```python
from build123d import *

# Parameters (mm, degrees)
SKETCH_1_W                   = 80
SKETCH_1_H                   = 40
EXTRUDE_1_DEPTH              = 20
HOLE_WIZARD_M3_1_D           = 4
HOLE_WIZARD_M3_1_CBORE_D     = 7
HOLE_WIZARD_M3_1_CBORE_DEPTH = 7
SKETCH_6_W                   = 7
SKETCH_6_H                   = 24
EXTRUDE_2_DEPTH              = 19
CUT_EXTRUDE_1_REACH          = 76.973
SKETCH_7_R                   = 6
SKETCH_16_R                  = 1.6
CUT_EXTRUDE_2_DEPTH          = 39
CUT_EXTRUDE_3_DEPTH          = 6


with BuildPart() as part:
    # 草图1 → 凸台-拉伸1 (new body)
    with BuildSketch(Plane(origin=(0, 0, 0), x_dir=(1, 0, 0), z_dir=(0, 1, 0))):
        with Locations((40, -20)):
            Rectangle(SKETCH_1_W, SKETCH_1_H)
    extrude(amount=EXTRUDE_1_DEPTH)

    # M3 六角圆柱头螺钉的柱形沉头孔1 (through all)
    with Locations(Plane(origin=(0, 0, 0), x_dir=(-1, 0, 0), z_dir=(0, -1, 0))):
        with Locations((-4, -4), (-4, -17.5), (-4, -28), (-28, -4)):
            CounterBoreHole(HOLE_WIZARD_M3_1_D / 2, HOLE_WIZARD_M3_1_CBORE_D / 2, HOLE_WIZARD_M3_1_CBORE_DEPTH)

    # 草图6 → 凸台-拉伸2 (add)
    with BuildSketch(Plane(origin=(0, 20, 0), x_dir=(1, 0, 0), z_dir=(0, 1, 0))):
        with Locations((53.5, -28)):
            Rectangle(SKETCH_6_W, SKETCH_6_H)
        with Locations((76.5, -28)):
            Rectangle(SKETCH_6_W, SKETCH_6_H)
    extrude(amount=EXTRUDE_2_DEPTH)

    # 切除-拉伸1: up to this face of the body (flat: up to its plane)
    cut_extrude_1_end = Plane(part.part.faces().sort_by_distance((80, 17.079617834, 22.904458599))[0])
    # 草图7 → 切除-拉伸1 (cut, up to the picked face)
    with BuildSketch(Plane.ZY.offset(-50), mode=Mode.PRIVATE) as cut_extrude_1_sk1:
        with Locations((28, 39)):
            Circle(SKETCH_7_R)
    cut_extrude_1_tool1 = split(extrude(cut_extrude_1_sk1.sketch, amount=-CUT_EXTRUDE_1_REACH, mode=Mode.PRIVATE), bisect_by=cut_extrude_1_end, keep=Keep.BOTH, mode=Mode.PRIVATE)
    add(cut_extrude_1_tool1.solids().sort_by(Axis((50, 39, 28), (1, 0, 0)))[0], mode=Mode.SUBTRACT)

    # 草图16 → 切除-拉伸2 (cut)
    with BuildSketch(Plane(origin=(0, 39, 0), x_dir=(1, 0, 0), z_dir=(0, 1, 0))):
        with Locations(Location((53.5, -37, 0), (0, 0, 270))):
            Circle(SKETCH_16_R)
        with Locations(Location((53.5, -19, 0), (0, 0, 270))):
            Circle(SKETCH_16_R)
        with Locations(Location((76.5, -19, 0), (0, 0, 270))):
            Circle(SKETCH_16_R)
        with Locations(Location((76.5, -37, 0), (0, 0, 270))):
            Circle(SKETCH_16_R)
    extrude(amount=-CUT_EXTRUDE_2_DEPTH, mode=Mode.SUBTRACT)

    # 草图17 → 切除-拉伸3 (cut)
    with BuildSketch(Plane.XZ):
        Polygon((56.733161507, 37), (55.116580754, 39.8), (51.883419246, 39.8), (50.266838493, 37), (51.883419246, 34.2), (55.116580754, 34.2), align=None)
        Polygon((73.266843837, 37.005878434), (74.878331045, 34.202943845), (78.111487208, 34.197065411), (79.733156163, 36.994121566), (78.121668955, 39.797056155), (74.888512792, 39.802934589), align=None)
        Polygon((56.733161283, 18.998795225), (55.117624008, 21.799397418), (51.884462725, 21.800602193), (50.266838717, 19.001204775), (51.882375992, 16.200602582), (55.115537275, 16.199397807), align=None)
        Polygon((79.733152762, 18.992479982), (78.123088908, 21.796232417), (74.889936146, 21.803752435), (73.266847238, 19.007520018), (74.876911092, 16.203767583), (78.110063854, 16.196247565), align=None)
    extrude(amount=-CUT_EXTRUDE_3_DEPTH, mode=Mode.SUBTRACT)


solid = part.part
```
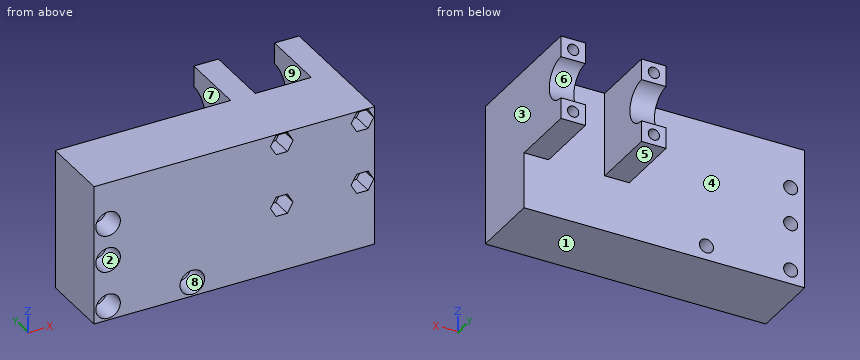
Design review of the part built by this model. Coordinates are the model's own, in mm. Face numbers are marked on the shaded views. A direction names the side the tool comes from. Give positions to 0.01 mm unless a question says otherwise; leave off trailing zeros. Order: outer loops, then holes, each group sorted by start corner. A loop starts at its lowest first (then second) coordinate and runs counter-clockwise, first axis right, second up. Notation, with made-up numbers: (-15, -32.5) - (31, -32.5) arc R22 cw to (31, 5.5) - close; hole circle Ø11 at (12, -5). An arc over 180 degrees is marked (long way). Use a Markdown table: item, result. Add a question column.
(1) Add section B-B on x = 28. Give the boundary of the cut face in (y, z).
(2) Mouldability with a two-part tool opening along X and no side actions: class the marked faces 1, 2, 3 and 4 as +X half, -X half, draft (parallel to the pull), parting line (faces both ways), or undercut.
(3) Add section A-A on y = 29.5. Give the boundary of the cut face in (x, z), then the cut area to 3 significant figures.
(4) Clearance check with flat-ended pins moving along their axes: P1, Ø3.5, axis at x = 54, y = 33.5, coming from the -Z side; P2, Ø8, axis at x = 4, z = 28, coming from the +Y side; P3, Ø5, axis at x = 76.5, z = 19, coming from the -Y side; P4, Ø1.7, axis at x = 53, z = 36.5, coming from the -Y side. State where each tip first meets the part, or that it passes through.
(5) Add section C-C on y = 17.5. Give the number of separate pieces and of enclosed holes in the cut face, then the cut area to 3 significant figures.
(6) Machinability: for the marked faces 5, 6, 7, 8 and 9, which of the approach directions +Z, -Z, +X, -X, +Y, -Y give a long, thin tool a straight path to every point of the face, cutting with its end or side? Answer none if there is none.
(7) Wall thickness on probe 1 along X at (y, z) = (25.5, 37); probe 2 along X at (y, z) = (5.5, 17.5); probe 3 along X at (y, z) = (17, 37): over which ranges is each line inside the solid? List them lowest first. Write a range as [from, to].
(8) Add section D-D on x = 4. Give the boundary of the cut face in (y, z).
Report:
| question | item | result |
|---|---|---|
| 1 | outline | (0, 0) - (20, 0) - (20, 2) - (7, 2) - (7, 0.5) - (0, 0.5) - close; (0, 7.5) - (7, 7.5) - (7, 6) - (20, 6) - (20, 40) - (0, 40) - close |
| 2 | face 1 | draft |
| 2 | face 2 | undercut |
| 2 | face 3 | +X half |
| 2 | face 4 | undercut |
| 3 | outline | (50, 16) - (57, 16) - (57, 40) - (50, 40) - close; (73, 16) - (80, 16) - (80, 40) - (73, 40) - close; hole circle Ø3.2 at (53.5, 19); hole circle Ø3.2 at (53.5, 37); hole circle Ø3.2 at (76.5, 19); hole circle Ø3.2 at (76.5, 37) |
| 3 | area | 304 mm² |
| 4 | P1 | stops at z = 16 |
| 4 | P2 | stops at y = 20 |
| 4 | P3 | stops at y = 6 |
| 4 | P4 | passes through |
| 5 | separate pieces | 1 |
| 5 | enclosed holes | 8 |
| 5 | area | 3,120 mm² |
| 6 | face 5 | -Z, +X, -X, +Y |
| 6 | face 6 | +X, -X, +Y |
| 6 | face 7 | +Z, -Z, -X, +Y |
| 6 | face 8 | -Y |
| 6 | face 9 | +Z, -Z, +Y |
| 7 | probe 1 | x = [50, 51.9], [55.1, 57], [73, 74.9], [78.1, 80] |
| 7 | probe 2 | x = [0, 0.5], [7.5, 51.13], [55.87, 74.13], [78.87, 80] |
| 7 | probe 3 | x = [0, 51.9], [55.1, 74.9], [78.1, 80] |
| 8 | outline | (0, 0) - (20, 0) - (20, 2) - (7, 2) - (7, 0.5) - (0, 0.5) - close; (0, 7.5) - (7, 7.5) - (7, 6) - (20, 6) - (20, 15.5) - (7, 15.5) - (7, 14) - (0, 14) - close; (0, 21) - (7, 21) - (7, 19.5) - (20, 19.5) - (20, 26) - (7, 26) - (7, 24.5) - (0, 24.5) - close; (0, 31.5) - (7, 31.5) - (7, 30) - (20, 30) - (20, 40) - (0, 40) - close |
